Check sheet for the modelled part. Datum: model origin and axes. Units: mm. Face numbers are marked on the shaded views. Round coordinates to 2 decimals unless told otherwise and drop trailing zeros. Order: outer loops, then holes, each group sorted by start corner. A loop starts at its lowest first (then second) coordinate and runs counter-clockwise, first axis right, second up.
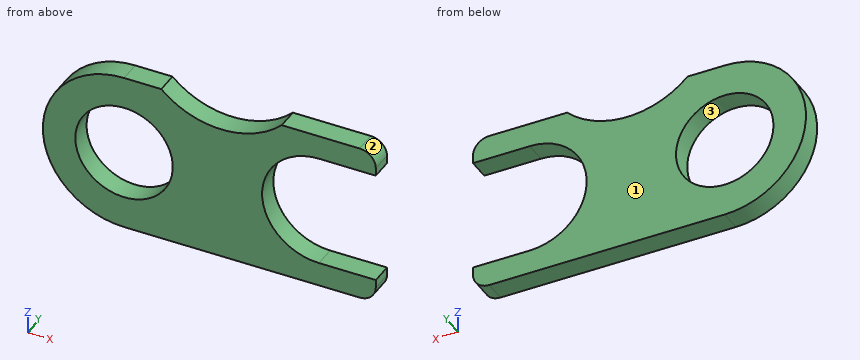
Autodesk Inventor part; units mm, degrees
ref_plane "YZ Plane" through (0, 0, 0) normal (1, 0, 0) x (0, 1, 0)
ref_plane "XZ Plane" through (0, 0, 0) normal (0, 1, 0) x (-1, 0, 0)
ref_plane "XY Plane" through (0, 0, 0) normal (0, 0, 1) x (1, 0, 0)
sketch "Skizze1" plane through (0, 0, 0) normal (0, 1, 0) x (-1, 0, 0)
  arc A0 (0, -7.5) -> (0, 7.5) centre (0, 0) ccw
  arc A1 (-18, -5.25) -> (-18, 5.25) centre (-18, 0) ccw
  line L0 (0, 7.5) -> (0, -7.5) construction
  line L1 (-18, 5.25) -> (-18, -5.25) construction
  line L2 (-18, 5.25) -> (-23.25, 5.25)
  line L3 (-18, -5.25) -> (-23.25, -5.25)
  line L4 (-23.25, 5.25) -> (-23.25, 6)
  line L5 (-23.25, -5.25) -> (-23.25, -6)
  line L6 (-21.75, -7.5) -> (0, -7.5)
  arc A2 (-21.75, 7.5) -> (-23.25, 6) centre (-21.75, 6) ccw
  arc A3 (-23.25, -6) -> (-21.75, -7.5) centre (-21.75, -6) ccw
  circle A4 centre (-18, 0) radius 5.25 construction
  circle A5 centre (0, 0) radius 4.5
  arc A6 (-14.5621, 7.5) -> (-3.4379, 7.5) centre (-9, 13.25) ccw
  line L7 (-21.75, 7.5) -> (-14.5621, 7.5)
  line L8 (-3.4379, 7.5) -> (0, 7.5)
  point P0 (-23.25, 0)
  point P1 (-9, 5.25)
  dimension "d4" = 10.5
  dimension "d0" = 15
  dimension "d1" = 10.5
  dimension "d2" = 18
  dimension "d3" = 1.5
  dimension "d5" = 9
  dimension "d8" = 8
  dimension "d9" = 9
extrude "Extrusion1" add sketch "Skizze1" along normal mid plane 2
properties part number "205 part 3" material "Gold"
Item 1: Scan lines: line 1 along Z through (x, y) = (0, 0.4); line 2 along Z through (x, y) = (18, -0.5); line 3 along X through (y, z) = (-0.65, -3.5). Record each from-to range of solid material in increasing order.
Answer:
line 1: z = -7.5 to -4.5, 4.5 to 7.5
line 2: z = -7.5 to -5.25, 5.25 to 7.5
line 3: x = -6.63 to -2.83, 2.83 to 14.09
Item 2: Release check for a two-part mould opening along Z. For the marked faces 1, 2 and 3 record: released by +Z, released by -Z, zero draft, split by the parting line, or undercut.
Answer:
face 1: zero draft
face 2: released by +Z
face 3: undercut
Item 3: Sectioned sample at D-D (z = -6.5). Record the cut outline in (x, y).
Answer:
outline: (-3.74, -1) - (23.16, -1) - (23.16, 1) - (-3.74, 1) - close
Item 4: Go/stop test with a flat-tipped pin: P1, Ø8, axis at x = 19.5, z = -1, coming from the +Y side. Record where the tip stops, or that it passes through.
Answer:
P1: passes through
Item 5: Sectioned sample at C-C (x = 13.5). Record the cut outline in (y, z).
Answer:
outline: (-1, -7.5) - (1, -7.5) - (1, -2.7) - (-1, -2.7) - close; (-1, 2.7) - (1, 2.7) - (1, 6.64) - (-1, 6.64) - close
Item 6: Sectioned sample at B-B (z = 0). Record the cut outline in (x, y).
Answer:
outline: (-7.5, -1) - (-4.5, -1) - (-4.5, 1) - (-7.5, 1) - close; (4.5, -1) - (12.75, -1) - (12.75, 1) - (4.5, 1) - close
Item 7: Sectioned sample at A-A (y = 0.7). Record the cut outline in (x, z).
Answer:
outline: (0, -7.5) - (21.75, -7.5) arc R1.5 ccw to (23.25, -6) - (23.25, -5.25) - (18, -5.25) arc R5.25 cw to (18, 5.25) - (23.25, 5.25) - (23.25, 6) arc R1.5 ccw to (21.75, 7.5) - (14.56, 7.5) arc R8 cw to (3.44, 7.5) - (0, 7.5) arc R7.5 ccw to start; hole circle Ø9 at (0, 0)
